The listing builds one solid part. Answer for the finished solid, in the listing's coordinates (mm). A direction names the side the tool comes from. Give positions to 0.01 mm unless a question says otherwise; leave off trailing zeros. Write each loop counter-clockwise with the first axis right and the second up, starting at its lowest first coordinate (ties: lowest second). Pieces come first, ordered by that corner, then holes. Notation, with made-up numbers: M 63,57.25 L 120,57.25 A21 ccw 120,96.25 Z; hole C 81.5,-25.75 d7. An arc over 180 degrees is marked long. Answer as a JSON object with one key per item and string values.
```python
from build123d import *

# Parameters (mm, degrees)
M3_ALT_GEN_ALYAN_HAV_A_BA_L_K_R_VIDA_I_D           = 3.4
M3_ALT_GEN_ALYAN_HAV_A_BA_L_K_R_VIDA_I_CSINK_D     = 6.72
M3_ALT_GEN_ALYAN_HAV_A_BA_L_K_R_VIDA_I_CSINK_ANGLE = 90
DAIRESEL_KAPLAMA2_COUNT                            = 10


with BuildPart() as part:
    # Çizim1 → Döndür3 (revolve)
    with BuildSketch(Plane.XY, mode=Mode.PRIVATE) as d_nd_r3_sk:
        with BuildLine():
            Line((-26.6, 0.54574792), (-26.6, 10.54574792))
            Line((-26.6, 10.54574792), (-25.1, 10.54574792))
            Line((-25.1, 10.54574792), (-25.1, 18.94574792))
            ThreePointArc((-25.1, 18.94574792), (-30.108474042, 31.037273878), (-42.2, 36.04574792))
            Line((-42.2, 36.04574792), (-55.5, 36.04574792))
            ThreePointArc((-55.5, 36.04574792), (-60.449747468, 38.096000452), (-62.5, 43.04574792))
            Line((-62.5, 43.04574792), (-62.5, 59.129332396))
            Line((-62.5, 59.129332396), (-64, 59.129332396))
            Line((-64, 59.129332396), (-64, 67.129332396))
            Line((-64, 67.129332396), (-66, 67.129332396))
            Line((-66, 67.129332396), (-66, 57.129332396))
            Line((-66, 57.129332396), (-64.5, 57.129332396))
            Line((-64.5, 57.129332396), (-64.5, 33.04574792))
            Line((-64.5, 33.04574792), (-39.98, 33.04574792))
            ThreePointArc((-39.98, 33.04574792), (-31.57957144, 29.56617648), (-28.1, 21.16574792))
            Line((-28.1, 21.16574792), (-28.1, 0.54574792))
            Line((-28.1, 0.54574792), (-26.6, 0.54574792))
        make_face()
    revolve(d_nd_r3_sk.sketch.rotate(Axis((0, 0, 0), (0, 1, 0)), 270), axis=Axis((0, 0, 0), (0, 1, 0)))

    # M3 Altıgen Alyan Havşa Başlı Kör Vida İçin Havşa4 (through all)
    with Locations(Plane(origin=(8.5, 33.04574792, 50.5), x_dir=(0, 0, -1), z_dir=(0, -1, 0))):
        with Locations((0, 0)):
            m3_alt_gen_alyan_hav_a_ba_l_k_r_vida_i = CounterSinkHole(M3_ALT_GEN_ALYAN_HAV_A_BA_L_K_R_VIDA_I_D / 2, M3_ALT_GEN_ALYAN_HAV_A_BA_L_K_R_VIDA_I_CSINK_D / 2, counter_sink_angle=M3_ALT_GEN_ALYAN_HAV_A_BA_L_K_R_VIDA_I_CSINK_ANGLE)

    # Dairesel Kaplama2: M3 Altıgen Alyan Havşa Başlı Kör Vida İçin Havşa4 ×10 about axis
    dairesel_kaplama2_axis = Axis((0, 0, 0), (0, 1, 0))
    for i in range(1, DAIRESEL_KAPLAMA2_COUNT):
        add(m3_alt_gen_alyan_hav_a_ba_l_k_r_vida_i.rotate(dairesel_kaplama2_axis, i * 360 / DAIRESEL_KAPLAMA2_COUNT), mode=Mode.SUBTRACT)


solid = part.part
```
1. A cutting plane is placed at B-B, the plane y = 16. Give the vertices of the cut face in (x, z).
Verdict:
{"outline": "C 0,0 d56.2; hole C 0,0 d50.2"}
2. Flat-ended cylindrical pins translate along their axes: pin 1 (1.5 mm diameter, centred on x = 4.5, y = 7.5, fed in from -Z); pin 2 (2 mm diameter, centred on x = 8.5, z = 50.5, fed in from -Y); pin 3 (1.5 mm diameter, centred on x = -30.5, z = -39.5, fed in from -Y); pin 4 (3 mm diameter, centred on x = -0.5, y = 35.5, fed in from +Z). Find the tip coordinate at first contact, or state that the pin passes through.
Verdict:
{"pin 1": "stops at z = -27.85", "pin 2": "passes through", "pin 3": "stops at y = 33.05", "pin 4": "stops at z = 64.5"}
3. A cutting plane is placed at D-D, the plane y = 8. Give the vertices of the cut face in (x, z).
Verdict:
{"outline": "C 0,0 d56.2; hole C 0,0 d53.2"}
4. For faces 1 (the flat face through (28, 33.046, 30)), 2 (the cylindrical face through (7.47, 35.39, 49.15)), 3 (the cylindrical face through (62.48, 63.19, 13.87)), determine the directions among +Z, -Z, +X, -X, +Y, -Y from which every point of the face is accessible in a straight line to the end or side of a thin tool.
Verdict:
{"face 1": "-Y", "face 2": "+Y, -Y", "face 3": "+Y"}
5. A cutting plane is placed at C-C, the plane x = 8.5. Count the separate pieces of the cut face and the enclosed holes in it, plus the area to 3 significant figures.
Verdict:
{"separate pieces": "3", "enclosed holes": "0", "area": "487 mm2"}
6. The mould has two halves that part along Z. Classify faces 4 (the cylindrical face through (64.43, 62.06, 14.31)), 5 (the flat face through (-16, 10.546, -20)), 6 (the flat face through (-35, 67.129, -54)): released by +Z, released by -Z, zero draft, split by the parting line, or undercut.
Verdict:
{"face 4": "split by the parting line", "face 5": "undercut", "face 6": "zero draft"}
7. Consider line 1 along X through (y, z) = (53.5, 0); line 2 along Z through (x, y) = (-1, 10); line 3 along Y through (x, z) = (-36.5, 36). Determine where each line is inside the solid, lowest interval first.
Verdict:
{"line 1": "x = -64.5 to -62.5, 62.5 to 64.5", "line 2": "z = -28.08 to -26.58, 26.58 to 28.08", "line 3": "y = 33.05 to 36.05"}
